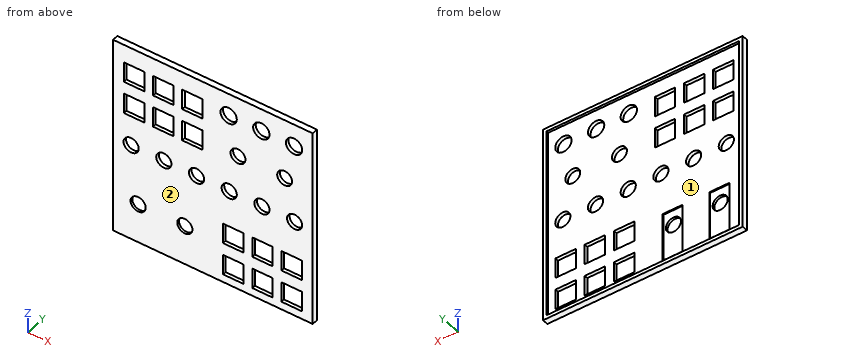
Autodesk Inventor part; units mm, degrees
ref_plane "YZ Plane" through (0, 0, 0) normal (1, 0, 0) x (0, 1, 0)
ref_plane "XZ Plane" through (0, 0, 0) normal (0, 1, 0) x (-1, 0, 0)
ref_plane "XY Plane" through (0, 0, 0) normal (0, 0, 1) x (1, 0, 0)
sketch "Sketch1" plane through (0, 0, 0) normal (0, 1, 0) x (-1, 0, 0)
  line L0 (0, 0) -> (-171, 0)
  line L1 (-171, 0) -> (-171, -171)
  line L2 (-171, -171) -> (0, -171)
  line L3 (0, -171) -> (0, 0)
  dimension "d0" = 171
  dimension "d1" = 171
extrude "Extrusion1" add sketch "Sketch1" along normal blind 3
sketch "Sketch2" plane through (0, 3, 0) normal (0, 1, 0) x (1, 0, 0)
  line L0 (171, 0) -> (171, 171)
  line L1 (171, 171) -> (0, 171)
  line L2 (0, 171) -> (0, 0)
  line L3 (0, 0) -> (171, 0)
  line L4 (3, 3) -> (3, 168)
  line L5 (3, 168) -> (168, 168)
  line L6 (168, 168) -> (168, 3)
  line L7 (168, 3) -> (3, 3)
  dimension "d98" = 165
extrude "Extrusion2" add sketch "Sketch2" along normal blind 2
sketch "Sketch3" plane through (0, 3, 0) normal (0, 1, 0) x (1, 0, 0)
  line L0 (3, 3) -> (168, 3) construction
  line L1 (168, 3) -> (168, 168) construction
  line L2 (168, 168) -> (3, 168) construction
  line L3 (3, 168) -> (3, 3) construction
  line L4 (4, 64) -> (82, 64) construction
  line L5 (82, 64) -> (82, 4) construction
  line L6 (82, 4) -> (4, 4) construction
  line L7 (4, 4) -> (4, 64) construction
  line L8 (89, 107) -> (167, 107) construction
  line L9 (167, 107) -> (167, 167) construction
  line L10 (167, 167) -> (89, 167) construction
  line L11 (89, 167) -> (89, 107) construction
  line L12 (4, 167) -> (79, 167) construction
  line L13 (79, 167) -> (79, 102) construction
  line L14 (4, 72) -> (4, 167) construction
  line L15 (4, 72) -> (167, 72) construction
  line L16 (167, 72) -> (167, 102) construction
  line L17 (167, 102) -> (79, 102) construction
  line L18 (87, 67) -> (167, 67) construction
  line L19 (167, 67) -> (167, 37) construction
  line L20 (167, 37) -> (87, 37) construction
  line L21 (87, 37) -> (87, 67) construction
  line L22 (87, 32) -> (167, 32) construction
  line L23 (167, 32) -> (167, 7) construction
  line L24 (167, 7) -> (87, 7) construction
  line L25 (87, 7) -> (87, 32) construction
  line L26 (9.25, 33.15) -> (26.75, 33.15)
  line L27 (26.75, 33.15) -> (26.75, 15.65)
  line L28 (26.75, 15.65) -> (9.25, 15.65)
  line L29 (9.25, 15.65) -> (9.25, 33.15)
  line L30 (9.25, 61.15) -> (26.75, 61.15)
  line L31 (9.25, 43.65) -> (9.25, 61.15)
  line L32 (26.75, 43.65) -> (9.25, 43.65)
  line L33 (26.75, 61.15) -> (26.75, 43.65)
  line L34 (34.25, 33.15) -> (51.75, 33.15)
  line L35 (34.25, 15.65) -> (34.25, 33.15)
  line L36 (51.75, 15.65) -> (34.25, 15.65)
  line L37 (51.75, 33.15) -> (51.75, 15.65)
  line L38 (34.25, 61.15) -> (51.75, 61.15)
  line L39 (34.25, 43.65) -> (34.25, 61.15)
  line L40 (51.75, 43.65) -> (34.25, 43.65)
  line L41 (51.75, 61.15) -> (51.75, 43.65)
  line L42 (59.25, 33.15) -> (76.75, 33.15)
  line L43 (59.25, 15.65) -> (59.25, 33.15)
  line L44 (76.75, 15.65) -> (59.25, 15.65)
  line L45 (76.75, 33.15) -> (76.75, 15.65)
  line L46 (59.25, 61.15) -> (76.75, 61.15)
  line L47 (59.25, 43.65) -> (59.25, 61.15)
  line L48 (76.75, 43.65) -> (59.25, 43.65)
  line L49 (76.75, 61.15) -> (76.75, 43.65)
  line L50 (9.25, 61.15) -> (9.25, 15.65) construction
  line L51 (9.25, 61.15) -> (76.75, 61.15) construction
  line L52 (94.25, 136.15) -> (111.75, 136.15)
  line L53 (111.75, 136.15) -> (111.75, 118.65)
  line L54 (111.75, 118.65) -> (94.25, 118.65)
  line L55 (94.25, 118.65) -> (94.25, 136.15)
  line L56 (94.25, 164.15) -> (111.75, 164.15)
  line L57 (94.25, 146.65) -> (94.25, 164.15)
  line L58 (111.75, 146.65) -> (94.25, 146.65)
  line L59 (111.75, 164.15) -> (111.75, 146.65)
  line L60 (119.25, 136.15) -> (136.75, 136.15)
  line L61 (119.25, 118.65) -> (119.25, 136.15)
  line L62 (136.75, 118.65) -> (119.25, 118.65)
  line L63 (136.75, 136.15) -> (136.75, 118.65)
  line L64 (119.25, 164.15) -> (136.75, 164.15)
  line L65 (119.25, 146.65) -> (119.25, 164.15)
  line L66 (136.75, 146.65) -> (119.25, 146.65)
  line L67 (136.75, 164.15) -> (136.75, 146.65)
  line L68 (144.25, 136.15) -> (161.75, 136.15)
  line L69 (144.25, 118.65) -> (144.25, 136.15)
  line L70 (161.75, 118.65) -> (144.25, 118.65)
  line L71 (161.75, 136.15) -> (161.75, 118.65)
  line L72 (144.25, 164.15) -> (161.75, 164.15)
  line L73 (144.25, 146.65) -> (144.25, 164.15)
  line L74 (161.75, 146.65) -> (144.25, 146.65)
  line L75 (161.75, 164.15) -> (161.75, 146.65)
  line L76 (94.25, 164.15) -> (94.25, 118.65) construction
  line L77 (94.25, 164.15) -> (161.75, 164.15) construction
  circle A0 centre (107, 52) radius 12.5 construction
  circle A1 centre (147, 52) radius 12.5 construction
  circle A2 centre (107, 52) radius 6.4
  circle A3 centre (147, 52) radius 6.4
  circle A4 centre (99, 19.5) radius 8.1 construction
  circle A5 centre (127, 19.5) radius 8.1 construction
  circle A6 centre (155, 19.5) radius 8.1 construction
  circle A7 centre (99, 19.5) radius 7
  circle A8 centre (127, 19.5) radius 7
  circle A9 centre (155, 19.5) radius 7
  circle A10 centre (155.5, 87) radius 6.5
  circle A11 centre (127.5, 87) radius 6.5
  circle A12 centre (99.5, 87) radius 6.5
  circle A13 centre (71.5, 87) radius 6.5
  circle A14 centre (43.5, 87) radius 6.5
  circle A15 centre (15.5, 87) radius 6.5
  circle A16 centre (61.5, 137) radius 6.5
  circle A17 centre (21.5, 137) radius 6.5
  point P0 (0, 0)
  point P1 (4, 34)
  point P2 (43, 61.15)
  point P3 (43, 64)
  point P4 (18, 43.65)
  point P5 (26.75, 52.4)
  point P6 (128, 164.15)
  point P7 (103, 146.65)
  point P8 (111.75, 155.4)
  point P9 (128, 164.15)
  point P10 (128, 107)
  point P11 (87, 52)
  point P12 (167, 19.5)
  point P13 (167, 87)
  point P14 (79, 134.5)
  point P15 (9.25, 24.4)
  point P16 (94.25, 127.4)
  dimension "d7" = 1
  dimension "d8" = 1
  dimension "d9" = 60
  dimension "d10" = 78
  dimension "d11" = 78
  dimension "d12" = 60
  dimension "d13" = 1
  dimension "d14" = 1
  dimension "d15" = 1
  dimension "d16" = 1
  dimension "d17" = 75
  dimension "d19" = 1
  dimension "d20" = 5
  dimension "d21" = 30
  dimension "d22" = 5
  dimension "d23" = 5
  dimension "d24" = 1
  dimension "d27" = 5
  dimension "d28" = 5
  dimension "d29" = 1
  dimension "d30" = 4
  dimension "d31" = 25
  dimension "d32" = 17.5
  dimension "d33" = 17.5
  dimension "d37" = 28
  dimension "d40" = 25
  dimension "d44" = 5.25
  dimension "d45" = 2.85
  dimension "d46" = 14
  dimension "d47" = 11.6
  dimension "d52" = 17.5
  dimension "d53" = 17.5
  dimension "d54" = 28
  dimension "d55" = 25
  dimension "d57" = 30
  dimension "d58" = 80
  dimension "d59" = 25
  dimension "d60" = 25
  dimension "d61" = 20
  dimension "d62" = 40
  dimension "d63" = 12.8
  dimension "d64" = 12.8
  dimension "d67" = 80
  dimension "d68" = 16.2
  dimension "d69" = 16.2
  dimension "d70" = 16.2
  dimension "d71" = 28
  dimension "d72" = 28
  dimension "d73" = 12
  dimension "d74" = 14
  dimension "d75" = 14
  dimension "d76" = 14
  dimension "d77" = 13
  dimension "d80" = 28
  dimension "d85" = 11.5
  dimension "d86" = 163
  dimension "d87" = 65
  dimension "d88" = 95
  dimension "d89" = 88
  dimension "d90" = 13
  dimension "d91" = 13
  dimension "d92" = 30
  dimension "d93" = 40
  dimension "d94" = 17.5
extrude "Extrusion3" cut sketch "Sketch3" against normal up to surface (3 mm away)
sketch "Sketch5" plane through (0, 3, 0) normal (0, 1, 0) x (1, 0, 0)
  circle A0 centre (21.5, 137) radius 6.5 construction
  circle A1 centre (61.5, 137) radius 6.5 construction
  line L0 (12.9, 165.8) -> (30.1, 165.8)
  line L1 (30.1, 165.8) -> (30.1, 124)
  line L2 (30.1, 124) -> (12.9, 124)
  line L3 (12.9, 124) -> (12.9, 165.8)
  line L4 (70.1, 124) -> (52.9, 124)
  line L5 (52.9, 124) -> (52.9, 165.8)
  line L6 (52.9, 165.8) -> (70.1, 165.8)
  line L7 (70.1, 165.8) -> (70.1, 124)
  point P0 (0, 0)
  point P1 (21.5, 165.8)
  point P2 (61.5, 165.8)
  point P3 (61.5, 124)
  point P4 (21.5, 124)
  dimension "d99" = 13
  dimension "d100" = 28.8
  dimension "d101" = 17.2
  dimension "d102" = 17.2
extrude "Extrusion5" cut sketch "Sketch5" against normal blind 1
equation "\"d8\" = d7"
equation "\"d11\" = d10"
equation "\"d12\" = d9"
equation "\"d13\" = d7"
equation "\"d14\" = d7"
equation "\"d15\" = d7"
equation "\"d16\" = d7"
equation "\"d19\" = d7"
equation "\"d24\" = d7"
equation "\"d29\" = d7"
equation "\"d60\" = d59"
equation "\"d61\" = -0.5 * d62 + 0.5 * d58"
equation "\"d64\" = d63"
equation "\"d69\" = d68"
equation "\"d70\" = d68"
equation "\"d72\" = d71"
equation "\"d73\" = -d71 + 0.5 * d67"
equation "\"d75\" = d74"
equation "\"d76\" = d74"
properties part number "Faceplate"
The model under review builds one solid part; all positions refer to its coordinate system, in mm. Face numbers are marked on the shaded views. Give positions to 0.01 mm unless a question says otherwise; leave off trailing zeros. Order: outer loops, then holes, each group sorted by start corner. A loop starts at its lowest first (then second) coordinate and runs counter-clockwise, first axis right, second up. Notation, with made-up numbers: M -25.75,0 L 6.25,0 A27 cw 6.25,36 Z; hole C -3.75,12 d5. An arc over 180 degrees is marked long. Answer in a Markdown table with one row per item. Add a question column.
1. Add section D-D on z = -160. State the section outline as (x, y) points.
2. For pin 1 Ø11.5 at (x, z) = (99.5, -87) entering from +Y; pin 2 Ø1 at (x, z) = (81.5, -62) entering from +Y; pin 3 Ø8.5 at (x, z) = (58, -136.5) entering from +Y, all flat-tipped, find the tip position at first contact; note any pin that passes through.
3. Add section C-C on z = -87. Count the separate pieces of the cut face and the enclosed holes in it, plus the area to 3 significant figures.
4. Add section B-B on y = 3.95. State the section outline as (x, z) points.
5. To check wall thickness, follow line 1 along X through (y, z) = (2.45, -151); line 2 along Z through (x, y) = (107, 1.4); line 3 along X through (y, z) = (1.65, -52). State the ranges of each line that lie inside material, in increasing order.
6. Add section A-A on x = 43.5. State the section outline as (y, z) points.
7. Mouldability with a two-part tool opening along Z and no side actions: class the marked faces 1 and 2 as released by +Z, released by -Z, zero draft, split by the parting line, or undercut.
The answers:
| question | item | result |
|---|---|---|
| 1 | outline | M 0,0 L 94.25,0 L 94.25,3 L 70.1,3 L 70.1,2 L 52.9,2 L 52.9,3 L 30.1,3 L 30.1,2 L 12.9,2 L 12.9,3 L 3,3 L 3,5 L 0,5 Z; M 111.75,0 L 119.25,0 L 119.25,3 L 111.75,3 Z; M 136.75,0 L 144.25,0 L 144.25,3 L 136.75,3 Z; M 161.75,0 L 171,0 L 171,5 L 168,5 L 168,3 L 161.75,3 Z |
| 2 | pin 1 | through |
| 2 | pin 2 | y = 3 |
| 2 | pin 3 | y = 2 |
| 3 | separate pieces | 7 |
| 3 | enclosed holes | 0 |
| 3 | area | 291 mm2 |
| 4 | outline | M 0,-171 L 171,-171 L 171,0 L 0,0 Z; hole M 3,-168 L 168,-168 L 168,-3 L 3,-3 Z |
| 5 | line 1 | 0 to 12.9, 30.1 to 52.9, 70.1 to 94.25, 111.75 to 119.25, 136.75 to 144.25, 161.75 to 171 |
| 5 | line 2 | -171 to -164.15, -146.65 to -136.15, -118.65 to -58.4, -45.6 to 0 |
| 5 | line 3 | 0 to 9.25, 26.75 to 34.25, 51.75 to 59.25, 76.75 to 100.6, 113.4 to 140.6, 153.4 to 171 |
| 6 | outline | M 0,-171 L 5,-171 L 5,-168 L 3,-168 L 3,-93.5 L 0,-93.5 Z; M 0,-80.5 L 3,-80.5 L 3,-61.15 L 0,-61.15 Z; M 0,-43.65 L 3,-43.65 L 3,-33.15 L 0,-33.15 Z; M 0,-15.65 L 3,-15.65 L 3,-3 L 5,-3 L 5,0 L 0,0 Z |
| 7 | face 1 | undercut |
| 7 | face 2 | zero draft |
